Job drawing, mm, ordinate dimensions from the low corner. One solid piece. A direction names the side the tool comes from. Give positions to 0.01 mm unless a question says otherwise; leave off trailing zeros. Order: outer loops, then holes, each group sorted by start corner. A loop starts at its lowest first (then second) coordinate and runs counter-clockwise, first axis right, second up.
Item 1: Band-saw the part on C-C on z = 131. Give the cut face in (x, y) (3 decimals), plus the area to 3 significant figures.
Item 2: Wall check: L1, parallel to X at y = 16.5, z = 67 (3 decimals); L2, parallel to Y at x = 74.85, z = 12.7; L3, parallel to Y at x = 21.5, z = 144 (3 decimals). Give the ranges that are in metal, low to high.
Item 3: Band-saw the part on B-B on x = 38.1. Give the cut face in (y, z) (3 decimals).
Item 4: Flat gauge pin, fed straight in: P1, Ø6.5, axis at y = 25.4, z = 12.7, coming from the -X side. Where does the tip first touch, or does it go through?
Item 5: Band-saw the part on D-D on y = 25.4. Give the cut face in (x, z) (3 decimals).
Item 6: Band-saw the part on A-A on y = 17.5. Give the cut face in (x, z) (3 decimals), plus the area to 3 significant figures.
Item 7: Which spindle directions (+Z, -Z, +X, -X, +Y, -Y) get a long thin tool onto all of the face, cutting with end or side? Do the marked faces 4 and 5. Say none if no direction does.
Item 8: Two-plate mould, pull along X, no slides. Class the marked faces 1, 2 and 3: released by +X, released by -X, zero draft, split by the parting line, or undercut.
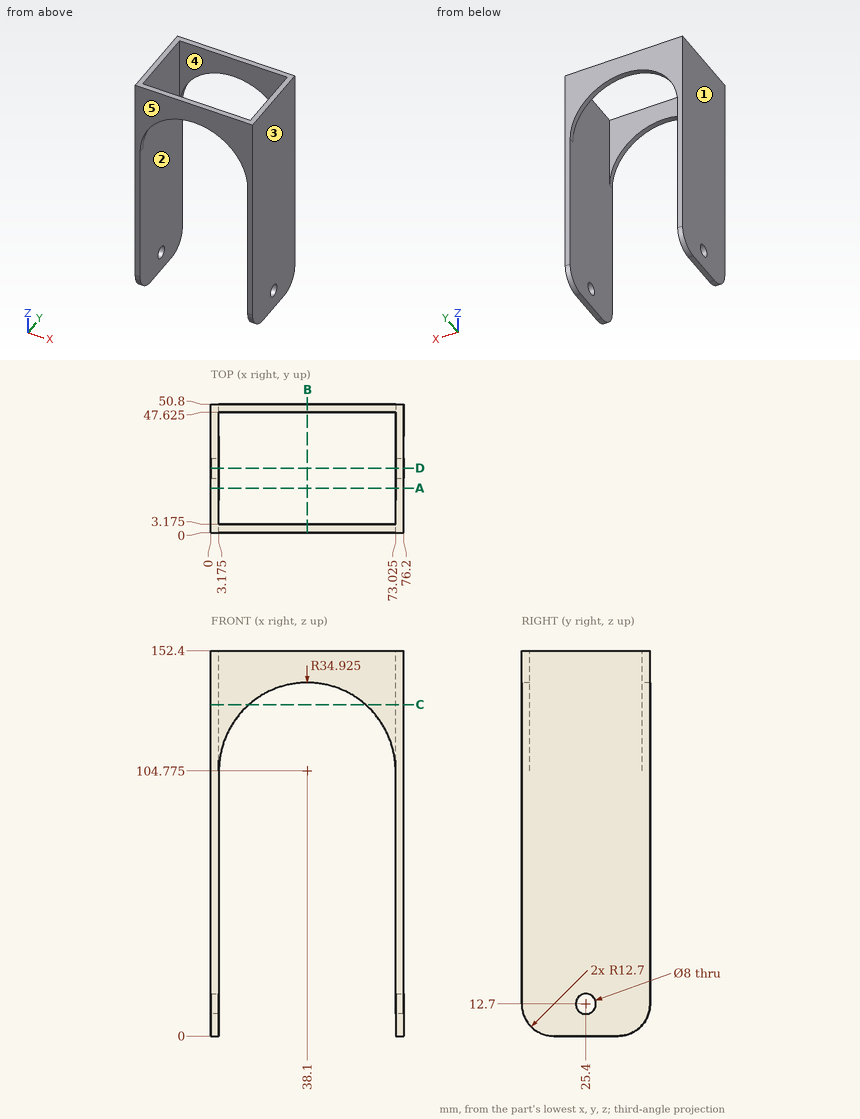
The answers:
1. outline: (0, 0) - (15.035, 0) - (15.035, 3.175) - (3.175, 3.175) - (3.175, 47.625) - (15.035, 47.625) - (15.035, 50.8) - (0, 50.8) - close; (61.165, 0) - (76.2, 0) - (76.2, 50.8) - (61.165, 50.8) - (61.165, 47.625) - (73.025, 47.625) - (73.025, 3.175) - (61.165, 3.175) - close
1. area: 473 mm2
2. L1: x = 0 to 3.175, 73.025 to 76.2
2. L2: y = 0 to 21.4, 29.4 to 50.8
2. L3: y = 0 to 3.175, 47.625 to 50.8
3. outline: (0, 139.7) - (3.175, 139.7) - (3.175, 152.4) - (0, 152.4) - close; (47.625, 139.7) - (50.8, 139.7) - (50.8, 152.4) - (47.625, 152.4) - close
4. P1: passes through
5. outline: (0, 0) - (3.175, 0) - (3.175, 8.7) - (0, 8.7) - close; (0, 16.7) - (3.175, 16.7) - (3.175, 152.4) - (0, 152.4) - close; (73.025, 0) - (76.2, 0) - (76.2, 8.7) - (73.025, 8.7) - close; (73.025, 16.7) - (76.2, 16.7) - (76.2, 152.4) - (73.025, 152.4) - close
6. outline: (0, 0) - (3.175, 0) - (3.175, 152.4) - (0, 152.4) - close; (73.025, 0) - (76.2, 0) - (76.2, 152.4) - (73.025, 152.4) - close
6. area: 968 mm2
7. face 4: +Z, -Z
7. face 5: +Z, -Z, +X, -X, -Y
8. face 1: released by -X
8. face 2: undercut
8. face 3: released by +X
